```python
from build123d import *

# Parameters (mm, degrees)
SKETCH1_R           = 2.25
SKETCH1_W           = 20
SKETCH1_H           = 40.5
BOSS_EXTRUDE1_DEPTH = 3


with BuildPart() as part:
    # Sketch1 → Boss-Extrude1 (new body)
    with BuildSketch(Plane.XY):
        with BuildLine():
            Line((-5, 44.75), (-5, -4.25))
            Line((-5, -4.25), (5.31559474, -65.676668518))
            ThreePointArc((5.31559474, -65.676668518), (10, -69.64), (14.68440526, -65.676668518))
            Line((14.68440526, -65.676668518), (25, -4.25))
            Line((25, -4.25), (25, 44.75))
            ThreePointArc((25, 44.75), (10, 59.75), (-5, 44.75))
        make_face()
        with Locations((14.75, -4.25)):
            Circle(SKETCH1_R, mode=Mode.SUBTRACT)
        with Locations((5.25, -4.25)):
            Circle(SKETCH1_R, mode=Mode.SUBTRACT)
        with Locations((14.75, 44.75)):
            Circle(SKETCH1_R, mode=Mode.SUBTRACT)
        with Locations((5.25, 44.75)):
            Circle(SKETCH1_R, mode=Mode.SUBTRACT)
        with Locations((10, 20.25)):
            Rectangle(SKETCH1_W, SKETCH1_H, mode=Mode.SUBTRACT)
    extrude(amount=BOSS_EXTRUDE1_DEPTH)


solid = part.part
```
CAD build for the part. Positions are in the model's coordinates, mm. A direction names the side the tool comes from. Coordinates: 2 decimals unless noted, no trailing zeros. Order: outer loops, then holes, each group sorted by start corner. A loop starts at its lowest first (then second) coordinate and runs counter-clockwise, first axis right, second up. Notation, with made-up numbers: M 20.25,8.25 L 57.25,8.25 A36 cw 57.25,47.25 Z; hole C 55,14.25 d10. An arc over 180 degrees is marked long. Write each question's results on one line, items separated by ' | '. Start each with the question number.
Q1. Cut at B-B (x = 10). List the corners of the cut face in (y, z), then the cut area to 3 significant figures.
Q2. Cut at C-C (z = 0.7). List the corners of the cut face in (x, y).
Q3. Flat gauge pins, fed straight in: P1, Ø3.5, axis at x = 5.25, y = -4.25, coming from the +Z side; P2, Ø1.5, axis at x = 5.5, z = 1, coming from the +Y side. Where does each tip first touch, or does it go through?
Q4. Pull direction X, two halves, no side cores. Call faces 1 (the flat face through (0, 20, 1)), 2 (the flat face through (0.086, -34.533, 1.479)), 3 (the cylindrical face through (9.91, -69.64, 1.48)): +X half, -X half, draft (parallel to the pull), parting line (faces both ways), or undercut.
Q5. Which spindle directions (+Z, -Z, +X, -X, +Y, -Y) get a long thin tool onto all of the face, cutting with end or side? Do faces 4 (the flat face through (-5, 21, 1)), 5 (the flat face through (20, 20, 1)). Say none if no direction does.
Q6. Drill centre lines: probe 1 along X at (y, z) = (0.5, 0.6); probe 2 along Y at (x, z) = (11, 0.4); probe 3 along Y at (x, z) = (11.5, 2.4). Where is each one in solid material? Low to high. Write a range as from..to.
Q7. Cut at A-A (y = 4). List the corners of the cut face in (x, z), then the cut area to 3 significant figures.
Found:
1) outline: M -69.64,0 L 0,0 L 0,3 L -69.64,3 Z; M 40.5,0 L 59.75,0 L 59.75,3 L 40.5,3 Z | area: 267 mm²
2) outline: M -5,-4.25 L 5.32,-65.68 A4.75 ccw 14.68,-65.68 L 25,-4.25 L 25,44.75 A15 ccw -5,44.75 Z; hole M 0,0 L 20,0 L 20,40.5 L 0,40.5 Z; hole C 5.25,-4.25 d4.5; hole C 5.25,44.75 d4.5; hole C 14.75,-4.25 d4.5; hole C 14.75,44.75 d4.5
3) P1: through | P2: y = 59.27
4) face 1: undercut | face 2: -X half | face 3: parting line
5) face 4: +Z, -Z, -X, +Y, -Y | face 5: +Z, -Z
6) probe 1: -5..0, 20..25 | probe 2: -69.53..0, 40.5..59.72 | probe 3: -69.4..0, 40.5..59.67
7) outline: M -5,0 L 0,0 L 0,3 L -5,3 Z; M 20,0 L 25,0 L 25,3 L 20,3 Z | area: 30.0 mm²
